Input: part model. Units: mm. Frame: model coordinates. Face numbers are marked on the shaded views. A direction names the side the tool comes from. Give positions to 0.01 mm unless a question says otherwise; leave off trailing zeros. Loops run counter-clockwise (first coordinate to the right, second up) from the corner with the lowest first, then second, coordinate; pieces in that order, holes last. Notation, with made-up numbers: (-34.75, -19.5) -> (-9.75, -19.5) arc R24 ccw to (-9.75, 19.5) -> close; hole circle Ø11 at (88, 33.25). An arc over 180 degrees is marked (long way). Answer as a JSON object with one key per item and string values.
```python
from build123d import *

# Parameters (mm, degrees)
CUT_EXTRUDE1_DEPTH      = 5.816666667
CUT_EXTRUDE1_DEPTH_BACK = 10
SKETCH3_R               = 2.75
CUT_EXTRUDE2_DEPTH      = 3.0000001
CUT_EXTRUDE2_DEPTH_BACK = 7.0000001


with BuildPart() as part:
    # Sketch1 → Revolve1 (revolve)
    with BuildSketch(Plane.XY):
        with BuildLine():
            Line((0, 0), (0, 44))
            Line((0, 44), (-2, 44))
            Line((-2, 44), (-2, 0))
            Line((-2, 0), (-4, 0))
            Line((-4, 0), (-4, -11.5))
            ThreePointArc((-4, -11.5), (-4.25, -16.45), (0, -19))
            Line((0, -19), (0, 0))
        make_face()
    revolve(axis=Axis((0, 0, 0), (0, 1, 0)))

    # Sketch2 → Cut-Extrude1 (cut, two sides)
    with BuildSketch(Plane(origin=(0, 0, 0), x_dir=(0, 0, -1), z_dir=(1, 0, 0))) as cut_extrude1_sk:
        with BuildLine():
            ThreePointArc((-2, -8.5), (-2.881966011, -7.763932023), (-4, -7.5))
            Line((-4, -7.5), (-4, -8.077978136))
            ThreePointArc((-4, -8.077978136), (-6.041123222, -13.901532194), (-2, -18.56514549))
            Line((-2, -18.56514549), (-2, -11.5))
            Line((-2, -11.5), (-2, -8.5))
        make_face()
        with BuildLine():
            Line((4, -8.077978136), (4, -7.5))
            ThreePointArc((4, -7.5), (2.881966011, -7.763932023), (2, -8.5))
            Line((2, -8.5), (2, -11.5))
            Line((2, -11.5), (2, -18.56514549))
            ThreePointArc((2, -18.56514549), (6.041123222, -13.901532194), (4, -8.077978136))
        make_face()
    extrude(amount=CUT_EXTRUDE1_DEPTH, mode=Mode.SUBTRACT)
    extrude(cut_extrude1_sk.sketch, amount=-CUT_EXTRUDE1_DEPTH_BACK, mode=Mode.SUBTRACT)

    # Sketch3 → Cut-Extrude2 (cut, two sides)
    with BuildSketch(Plane.XY.offset(2)) as cut_extrude2_sk:
        with Locations((0, -14)):
            Circle(SKETCH3_R)
    extrude(amount=CUT_EXTRUDE2_DEPTH, mode=Mode.SUBTRACT)
    extrude(cut_extrude2_sk.sketch, amount=-CUT_EXTRUDE2_DEPTH_BACK, mode=Mode.SUBTRACT)


solid = part.part
```
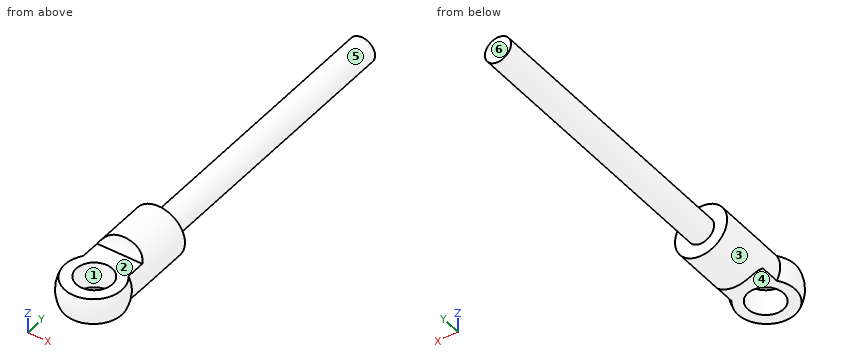
Q1. Section D-D, the plane y = -6. Return the cut outline in (x, z), then the cut area to 3 significant figures.
Evaluation:
{"outline": "circle Ø8 at (0, 0)", "area": "50.3 mm2"}
Q2. Pin query (flat end, axial travel): pin 1 (3 mm diameter, centred on x = 1.5, z = 1, fed in from -Y); pin 2 (2 mm diameter, centred on y = 24, z = 0, fed in from -X); pin 3 (2 mm diameter, centred on x = -0.5, y = 16, fed in from +Z). Return the tip coordinate at first contact, or that it passes through.
Evaluation:
{"pin 1": "stops at y = -18.99", "pin 2": "stops at x = -2", "pin 3": "stops at z = 2"}
Q3. Section B-B, the plane y = -14. Return the cut outline in (x, z).
Evaluation:
{"outline": "(-4.38, -2) -> (-2.75, -2) -> (-2.75, 2) -> (-4.38, 2) arc R4.81 ccw to start; (2.75, -2) -> (4.38, -2) arc R4.81 ccw to (4.38, 2) -> (2.75, 2) -> close"}
Q4. Section A-A, the plane x = 0. Return the cut outline in (y, z), then the cut area to 3 significant figures.
Evaluation:
{"outline": "(-18.57, -2) -> (-16.75, -2) -> (-16.75, 2) -> (-18.57, 2) arc R4.82 ccw to start; (-11.25, -2) -> (-8.5, -2) arc R2.5 cw to (-7.5, -4) -> (0, -4) -> (0, -2) -> (44, -2) -> (44, 2) -> (0, 2) -> (0, 4) -> (-7.5, 4) arc R2.5 cw to (-8.5, 2) -> (-11.25, 2) -> close", "area": "261 mm2"}
Q5. Draft query along X for the marked faces 1, 2 and 3. Return one class per face: +X half, -X half, draft (parallel to the pull), parting line (faces both ways), or undercut.
Evaluation:
{"face 1": "undercut", "face 2": "draft", "face 3": "parting line"}
Q6. Access query for the marked faces 4, 5 and 6. Directions: +Z, -Z, +X, -X, +Y, -Y. A direction counts if a zero-diameter tool reaches every point of the face in a straight line with its end or side. Return the directions, or none.
Evaluation:
{"face 4": "-Z, +X, -X, -Y", "face 5": "+Y", "face 6": "+Z, -Z, +X, -X, +Y"}
Q7. Section C-C, the plane y = 11.5. Return the cut outline in (x, z).
Evaluation:
{"outline": "circle Ø4 at (0, 0)"}
Q8. Ray query, line 1 along Y through (x, z) = (0, 0.85); line 2 along Y through (x, z) = (0, 0.55); line 3 along Z through (x, y) = (1.75, 10). Return the intervals inside material, ascending.
Evaluation:
{"line 1": "y = -18.92 to -16.75, -11.25 to 44", "line 2": "y = -18.97 to -16.75, -11.25 to 44", "line 3": "z = -0.97 to 0.97"}
